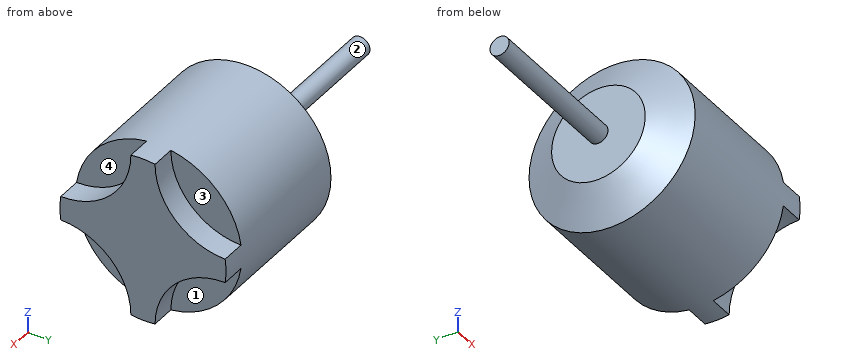
from build123d import *

# Parameters (mm, degrees)
SKETCH1_R            = 13.75
BOSS_EXTRUDE1_DEPTH  = 30
SKETCH2_R            = 1.585
BOSS_EXTRUDE2_DEPTH  = 25
CHAMFER1_SIZE        = 6
CHAMFER1_SIZE2       = 3.464101615
CUT_EXTRUDE1_START   = -4
CUT_EXTRUDE1_DEPTH   = 4
MIRROR2_START        = -4
MIRROR2_COPY_1_DEPTH = 4


with BuildPart() as part:
    # Sketch1 → Boss-Extrude1 (new body)
    with BuildSketch(Plane(origin=(0, 0, 0), x_dir=(0, 0, -1), z_dir=(1, 0, 0))):
        Circle(SKETCH1_R)
    extrude(amount=BOSS_EXTRUDE1_DEPTH)

    # Sketch2 → Boss-Extrude2 (add)
    with BuildSketch(Plane.ZY):
        with Locations(Location((0, 0, 0), (0, 0, 180))):
            Circle(SKETCH2_R)
    extrude(amount=BOSS_EXTRUDE2_DEPTH)

    # Chamfer1
    chamfer1_edges = [part.edges().sort_by_distance(p)[0] for p in [
        (0, 0, 13.75),
    ]]
    chamfer1_side = [part.faces().sort_by_distance(p)[0] for p in [
        (0, 0, 13.36109127),
    ]]
    chamfer(chamfer1_edges, length=CHAMFER1_SIZE, length2=CHAMFER1_SIZE2, reference=chamfer1_side[0])

    # Sketch3 → Cut-Extrude1 (cut)
    with BuildSketch(Plane(origin=(30, 0, 0), x_dir=(0, 0, -1), z_dir=(1, 0, 0)).offset(CUT_EXTRUDE1_START)):
        with BuildLine():
            ThreePointArc((-2, 13.60376786), (-5.398664919, 5.398664919), (-13.60376786, 2))
            ThreePointArc((-13.60376786, 2), (-9.722718241, 9.722718241), (-2, 13.60376786))
        make_face()
    cut_extrude1 = extrude(amount=CUT_EXTRUDE1_DEPTH, mode=Mode.SUBTRACT)

    # Mirror1: Cut-Extrude1 across plane
    add(cut_extrude1.mirror(Plane.XY), mode=Mode.SUBTRACT)

    # Mirror2: Cut-Extrude1 across plane
    add(cut_extrude1.mirror(Plane.ZX), mode=Mode.SUBTRACT)

    # Mirror2 copy 1 sketch → Mirror2 copy 1 (cut)
    with BuildSketch(Plane(origin=(30, 0, 0), x_dir=(0, 0, 1), z_dir=(1, 0, 0)).offset(MIRROR2_START)):
        with BuildLine():
            ThreePointArc((-2, 13.60376786), (-5.398664919, 5.398664919), (-13.60376786, 2))
            ThreePointArc((-13.60376786, 2), (-9.722718241, 9.722718241), (-2, 13.60376786))
        make_face()
    extrude(amount=MIRROR2_COPY_1_DEPTH, mode=Mode.SUBTRACT)


solid = part.part
Could you check a few things on this model? Use its own coordinates, in mm. Face numbers are marked on the shaded views. A direction names the side the tool comes from. Give positions to 0.01 mm unless a question says otherwise; leave off trailing zeros. Order: outer loops, then holes, each group sorted by start corner. A loop starts at its lowest first (then second) coordinate and runs counter-clockwise, first axis right, second up. Notation, with made-up numbers: (18.5, 80) - (60.5, 80) arc R26 cw to (60.5, 110) - close; hole circle Ø8 at (-29.5, 19.5). An arc over 180 degrees is marked (long way). One line per question, with ' | ' between items. Start each with the question number.
Item 1: I want a section at A-A on y = 0. Write out the boundary of the cut face in (x, z) (3 decimals).
Item 2: I need wall thicknesses on probe 1 along X at (y, z) = (1.75, 6); probe 2 along Y at (x, z) = (19.5, -1); probe 3 along Z at (x, y) = (2, -5.25). Which ranges of each line are inside material? Lowest first, please. Write a range as [from, to].
Item 3: I'm going to push flat-ended pins straight in: pin 1 Ø4 at (y, z) = (-8.5, 10.5) entering from -X; pin 2 Ø5 at (x, z) = (-9, 1) entering from +Y (3 decimals); pin 3 Ø6 at (y, z) = (-7.5, 5.5) entering from -X. Where does each tip first touch, or does it pass through?
Item 4: For the marked faces 1, 2, 3 and 4, which set-ups out of +Z, -Z, +X, -X, +Y, -Y let a thin tool reach every point of the face, with its end or its side?
Item 5: I want a section at D-D on x = -7.5. Write out the boundary of the cut face in (y, z) (3 decimals), then the cut area to 3 significant figures.
Item 6: I want a section at C-C on x = 8. Write out the boundary of the cut face in (y, z).
Verdict:
1) outline: (-25, -1.585) - (0, -1.585) - (0, -7.75) - (3.464, -13.75) - (30, -13.75) - (30, 13.75) - (3.464, 13.75) - (0, 7.75) - (0, 1.585) - (-25, 1.585) - close
2) probe 1: [0, 30] | probe 2: [-13.71, 13.71] | probe 3: [-9.91, 9.91]
3) pin 1: x = 2.17 | pin 2: y = 1.585 | pin 3: x = 0
4) face 1: -Z, +X, +Y | face 2: -X | face 3: +Z, +X, +Y | face 4: +Z, +X, -Y
5) outline: circle Ø3.17 at (0, 0) | area: 7.89 mm^2
6) outline: circle Ø27.5 at (0, 0)
